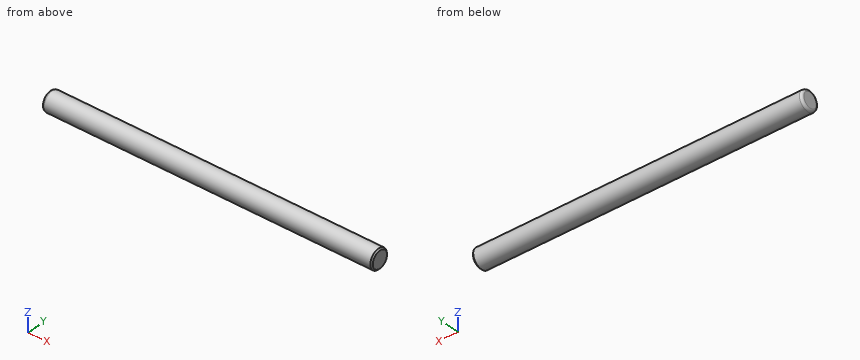
```python
from build123d import *

# Parameters (mm, degrees)
SCHNITT_LINEAR_AUSTRAGEN1_DEPTH      = 1001.015999872
SCHNITT_LINEAR_AUSTRAGEN1_DEPTH_BACK = 1001.015999872
SKIZZE2_W                            = 870
SKIZZE2_H                            = 18
VERRUNDUNG1_R                        = 1


with BuildPart() as part:
    # Skizze1 → Rotation1 (revolve)
    with BuildSketch(Plane.XY, mode=Mode.PRIVATE) as rotation1_sk:
        Polygon((0, 3.45875), (0, 0), (1000, 0), (1000, 3.45875), (999.45875, 4), (0.54125, 4), align=None)
    revolve(rotation1_sk.sketch.rotate(Axis((0, 0, 0), (1, 0, 0)), 270), axis=Axis((0, 0, 0), (1, 0, 0)))

    # Skizze2 → Schnitt-Linear austragen1 (cut, two sides: drawn at the far end of the back side and taken through both)
    with BuildSketch(Plane.XY.offset(-SCHNITT_LINEAR_AUSTRAGEN1_DEPTH_BACK)):
        with Locations((430, 0)):
            Rectangle(SKIZZE2_W, SKIZZE2_H)
    extrude(amount=SCHNITT_LINEAR_AUSTRAGEN1_DEPTH + SCHNITT_LINEAR_AUSTRAGEN1_DEPTH_BACK, mode=Mode.SUBTRACT)

    # Verrundung1
    verrundung1_edges = [part.edges().sort_by_distance(p)[0] for p in [
        (865, 0, 4),
    ]]
    fillet(verrundung1_edges, radius=VERRUNDUNG1_R)


solid = part.part
```
For this review, take the finished solid that the model builds, in its own axes (mm). Give positions to 0.01 mm unless a question says otherwise; leave off trailing zeros. Loops run counter-clockwise (first coordinate to the right, second up) from the corner with the lowest first, then second, coordinate; pieces in that order, holes last. Notation, with made-up numbers: M 22,15 L 45,15 A14 cw 45,37 Z; hole C 23.25,-30 d10. An arc over 180 degrees is marked long. One line per item, written item: value. Start each with the question number.
Q1. For L1, parallel to Z at x = 950, y = -2; L2, parallel to X at y = -0.75, z = 3; L3, parallel to Z at x = 942, y = -0.75, list the stretches that pass through material, from the lowest coordinate up.
Q2. Clearance check with flat-ended pins moving along their axes: pin 1 Ø1.5 at (x, y) = (901, 3) entering from -Z; pin 2 Ø3 at (x, y) = (941, -3) entering from +Z. State where each tip first meets the part, or that it passes through.
Q3. Add section A-A (x = 965). Give the boundary of the cut face in (y, z).
Reply:
1. L1: -3.46 to 3.46
1. L2: 865 to 1000
1. L3: -3.93 to 3.93
2. pin 1: z = -3.31
2. pin 2: z = 3.71
3. outline: C 0,0 d8
